from build123d import *

# Parameters (mm, degrees)
BOX001_W     = 10
BOX001_H     = 10
BOX001_DEPTH = 10
BOX_W        = 10
BOX_H        = 20
BOX_DEPTH    = 14


with BuildPart() as box001:
    # Box001 → Box001 (new body)
    with BuildSketch(Plane(origin=(10, 0, 0), x_dir=(1, 0, 0), z_dir=(0, 0, 1))):
        with Locations((5, 5)):
            Rectangle(BOX001_W, BOX001_H)
    extrude(amount=BOX001_DEPTH)


with BuildPart() as fusion:
    # Box → Box (new body)
    with BuildSketch(Plane.XY):
        with Locations((5, 10)):
            Rectangle(BOX_W, BOX_H)
    extrude(amount=BOX_DEPTH)

    # Fusion: union Box001
    add(box001.part)


solid = fusion.part
Source: CAD feature listing. Evaluate the final solid. Frame: model axes, mm. A direction names the side the tool comes from. Coordinates: 2 decimals unless noted, no trailing zeros. Loops run counter-clockwise (first coordinate to the right, second up) from the corner with the lowest first, then second, coordinate; pieces in that order, holes last. Notation, with made-up numbers: (-7, 63.5) - (27, 63.5) arc R24 cw to (27, 82.5) - close; hole circle Ø3 at (10, 65.25). An arc over 180 degrees is marked (long way). Return JSON: item names as keys, results as strings.
Q1. Section B-B, the plane y = 8.5. Return loops of the section in (x, z).
Results:
{"outline": "(0, 0) - (20, 0) - (20, 10) - (10, 10) - (10, 14) - (0, 14) - close"}
Q2. Section C-C, the plane x = 14.25. Return loops of the section in (y, z).
Results:
{"outline": "(0, 0) - (10, 0) - (10, 10) - (0, 10) - close"}
Q3. Access query for faces 1 (the flat face through (15, 10, 5)), 2 (the flat face through (5, 20, 7)), 3 (the flat face through (15, 5, 10)). Directions: +Z, -Z, +X, -X, +Y, -Y. A direction counts if a zero-diameter tool reaches every point of the face in a straight line with its end or side. Return the directions, or none.
Results:
{"face 1": "+Z, -Z, +X, +Y", "face 2": "+Z, -Z, +X, -X, +Y", "face 3": "+Z, +X, +Y, -Y"}
Q4. Section A-A, the plane z = 8. Return loops of the section in (x, y), plus the area to 3 significant figures.
Results:
{"outline": "(0, 0) - (20, 0) - (20, 10) - (10, 10) - (10, 20) - (0, 20) - close", "area": "300 mm2"}
Q5. Section D-D, the plane z = 11.25. Return loops of the section in (x, y).
Results:
{"outline": "(0, 0) - (10, 0) - (10, 20) - (0, 20) - close"}
Q6. Contact query for flat-ended pins moving along their axis: P1, Ø8, axis at y = 15.5, z = 5.5, coming from the -X side; P2, Ø3, axis at x = 13.5, z = 6.5, coming from the +Y side; P3, Ø11, axis at x = 17, y = 7, coming from the +Z side. Output: stop coordinate, or through.
Results:
{"P1": "x = 0", "P2": "y = 10", "P3": "z = 10"}
Q7. Material intervals for line 1 along X through (y, z) = (19, 6), sorted ascending.
Results:
{"line 1": "0 to 10"}
